Autodesk Inventor part; units mm, degrees
ref_plane "XZ Plane" through (0, 0, 0) normal (0, 1, 0) x (-1, 0, 0)
ref_plane "XY Plane" through (0, 0, 0) normal (0, 0, 1) x (1, 0, 0)
sketch "Sketch1" plane through (0, 0, 0) normal (1, 0, 0) x (0, 1, 0)
  line L0 (0, 0) -> (50, 0)
  line L1 (0, 5.25) -> (0, 12.5)
  line L2 (0, 12.5) -> (30, 12.5)
  line L3 (30, 12.5) -> (30, 7.5)
  line L4 (30, 7.5) -> (35, 7.5)
  line L5 (35, 7.5) -> (35, 3)
  line L6 (35, 3) -> (30, 2.5)
  line L7 (30, 2.5) -> (30, 0)
  line L8 (28, 0) -> (28, 5.25)
  line L9 (28, 5.25) -> (0, 5.25)
  line L10 (0, -2.5) -> (0, 15)
  dimension "d0" = 50
  dimension "d2" = 25
  dimension "d3" = 10.5
  dimension "d4" = 5
  dimension "d5" = 6
  dimension "d6" = 15
  dimension "d7" = 30
  dimension "d8" = 35
  dimension "d9" = 28
revolve "Revolution1" add sketch "Sketch1" angle 360 about axis through (0, 0, 0) along (0, 1, 0) contours L8 L9 L1 L2 L3 L4 L5 L6 L7 L0
ref_plane "Work Plane1" through (12.5, 15, 0) normal (1, 0, 0) x (0, 1, 0)
sketch "Sketch2" plane through (12.5, 15, 0) normal (1, 0, 0) x (0, 1, 0)
  line L0 (-15, 0) -> (-0.1, 0)
  circle A0 centre (-0.1, 0) radius 3.4
  dimension "d11" = 14.9
  dimension "d12" = 6.8
extrude "Extrusion1" cut sketch "Sketch2" against normal through all
properties part number "StuurPotentiometerConnector2.0_3DPrint"
Work out the finished part from the listing and answer in its coordinate system (mm). A direction names the side the tool comes from. Give positions to 0.01 mm unless a question says otherwise; leave off trailing zeros. Order: outer loops, then holes, each group sorted by start corner. A loop starts at its lowest first (then second) coordinate and runs counter-clockwise, first axis right, second up. Notation, with made-up numbers: M 14,-24.5 L 60,-24.5 A26 ccw 60,3.5 Z; hole C 76,85 d7. An arc over 180 degrees is marked long. Return JSON: item names as keys, results as strings.
1) Section B-B, the plane x = 0 is taken. Write down the section's boundary in (y, z).
Resolved:
{"outline": "M 0,-12.5 L 30,-12.5 L 30,-7.5 L 35,-7.5 L 35,-3 L 30,-2.5 L 30,2.5 L 35,3 L 35,7.5 L 30,7.5 L 30,12.5 L 0,12.5 L 0,5.25 L 28,5.25 L 28,-5.25 L 0,-5.25 Z"}
2) Section A-A, the plane z = 0 is taken. Write down the section's boundary in (x, y).
Resolved:
{"outline": "M -12.5,0 L -5.25,0 L -5.25,11.5 L -12.5,11.5 Z; M -12.5,18.3 L -5.25,18.3 L -5.25,28 L 5.25,28 L 5.25,18.3 L 12.5,18.3 L 12.5,30 L 7.5,30 L 7.5,35 L 3,35 L 2.5,30 L -2.5,30 L -3,35 L -7.5,35 L -7.5,30 L -12.5,30 Z; M 5.25,0 L 12.5,0 L 12.5,11.5 L 5.25,11.5 Z"}
3) Section C-C, the plane y = 20 is taken. Write down the section's boundary in (x, z), plus the area to 3 significant figures.
Resolved:
{"outline": "C 0,0 d25; hole C 0,0 d10.5", "area": "404 mm^2"}
4) Section D-D, the plane x = 10 is taken. Write down the section's boundary in (y, z), plus the area to 3 significant figures.
Resolved:
{"outline": "M 0,-7.5 L 30,-7.5 L 30,7.5 L 0,7.5 Z; hole C 14.9,0 d6.8", "area": "414 mm^2"}
5) A tool of negligible diameter and unlimited length cuts with its end or side. For faces 4 (the cylindrical face through (-8.191, 18.143, 1.021)), 5 (the flat face through (0, 30, 0)), 6 (the cylindrical face through (-3.55, 13.8, -3.87)), from which of +Z, -Z, +X, -X, +Y, -Y can it reach the whole face along a straight path? Write none if from no direction.
Resolved:
{"face 4": "+X, -X", "face 5": "+Y", "face 6": "-Y"}
6) Straight lines are drawn through the part: line 1 along Y through (x, z) = (8.5, 0); line 2 along X through (y, z) = (22, 0); line 3 along Y through (x, z) = (-2, 0.5). For each, find the intervals that lie inside material, in ascending order. Write a range as [from, to].
Resolved:
{"line 1": "[0, 11.5], [18.3, 30]", "line 2": "[-12.5, -5.25], [5.25, 12.5]", "line 3": "[28, 30]"}
7) Each of these flat-tipped pins is pushed along its axis until it touches: pin 1 (3 mm diameter, centred on x = 1.5, z = 0.5, fed in from -Y); pin 2 (4 mm diameter, centred on y = 14.9, z = 0, fed in from -X); pin 3 (1.5 mm diameter, centred on x = 6, y = 27, fed in from -Z); pin 4 (1 mm diameter, centred on x = -8.5, y = 17.5, fed in from -Z). Where does it stop, or does it pass through?
Resolved:
{"pin 1": "y = 28", "pin 2": "through", "pin 3": "z = -11.34", "pin 4": "z = -9.6"}
8) For a pull along Y with two mould halves and no side action, classify faces 1 (the flat face through (0, 28, 0)), 2 (the cylindrical face through (8.31, 18.143, 1.021)), 3 (the cylindrical face through (0.33, 32.535, -7.493)) as +Y half, -Y half, draft (parallel to the pull), parting line (faces both ways), or undercut.
Resolved:
{"face 1": "-Y half", "face 2": "undercut", "face 3": "draft"}
